Autodesk Inventor part; units mm, degrees
ref_plane "YZ Plane" through (0, 0, 0) normal (1, 0, 0) x (0, 1, 0)
ref_plane "XZ Plane" through (0, 0, 0) normal (0, 1, 0) x (-1, 0, 0)
ref_plane "XY Plane" through (0, 0, 0) normal (0, 0, 1) x (1, 0, 0)
sketch "Sketch1" plane through (0, 0, 0) normal (0, 0, 1) x (1, 0, 0)
  line L0 (-70, 0) -> (70, 0)
  line L1 (70, 0) -> (70, -400)
  line L2 (70, -400) -> (-70, -400)
  line L3 (-70, -400) -> (-70, 0)
  point P0 (0, 0)
  point P1 (0, 0)
  dimension "d0" = 140
  dimension "d1" = 400
extrude "Plate1" add sketch "Sketch1" along normal blind 2
sketch "Sketch2" plane through (72, -400, 2) normal (-1, 0, 0) x (0, -1, 0)
  line L0 (-400, 0) -> (0, 0)
  line L1 (0, 0) -> (0, -120)
  line L2 (0, -120) -> (-400, -120)
  line L3 (-400, -120) -> (-400, 0)
edge flange "Flange1" height 120 angle 90 thickness 2 bend radius 2.75 thickness toward (-1, 0, 0) relief round relief width 2 relief depth 1 edges at (70, -200, 0) wall of the first edge with corners at (72, 0, 2) (72, -400, 2) (72, -400, -118) (72, 0, -118)
bend "Bend1"
corner "Corner1"
sketch "Sketch3" plane through (-72, 0, 2) normal (1, 0, 0) x (0, 1, 0)
  line L0 (-400, 0) -> (0, 0)
  line L1 (0, 0) -> (0, -120)
  line L2 (0, -120) -> (-400, -120)
  line L3 (-400, -120) -> (-400, 0)
edge flange "Flange2" height 120 angle 90 thickness 2 bend radius 2.75 thickness toward (1, 0, 0) relief round relief width 2 relief depth 1 edges at (-70, -200, 0) wall of the first edge with corners at (-72, -400, 2) (-72, 0, 2) (-72, 0, -118) (-72, -400, -118)
bend "Bend2"
corner "Corner2"
sketch "Sketch4" plane through (70, 0, -120) normal (0, 0, 1) x (1, 0, 0)
  line L0 (0, -400) -> (0, 0)
  line L1 (0, 0) -> (25, 0)
  line L2 (25, 0) -> (25, -400)
  line L3 (25, -400) -> (0, -400)
edge flange "Flange3" height 25 angle 90 thickness 2 bend radius 2.75 thickness toward (0, 0, 1) relief round relief width 2 relief depth 1 edges at (72, -200, -118) wall of the first edge with corners at (70, -400, -120) (70, 0, -120) (95, 0, -120) (95, -400, -120)
bend "Bend3"
corner "Corner3"
sketch "Sketch5" plane through (-70, -400, -120) normal (0, 0, 1) x (1, 0, 0)
  line L0 (0, 400) -> (0, 0)
  line L1 (0, 0) -> (-25, 0)
  line L2 (-25, 0) -> (-25, 400)
  line L3 (-25, 400) -> (0, 400)
edge flange "Flange4" height 25 angle 90 thickness 2 bend radius 2.75 thickness toward (0, 0, 1) relief round relief width 2 relief depth 1 edges at (-72, -200, -118) wall of the first edge with corners at (-70, 0, -120) (-70, -400, -120) (-95, -400, -120) (-95, 0, -120)
bend "Bend4"
corner "Corner4"
sketch "Sketch6" plane through (95, -400, -118) normal (0, 0, 1) x (1, 0, 0)
  circle A0 centre (-10.125, 350) radius 4
  line L0 (-20.25, 400) -> (0, 400)
  point P0 (-95, 400)
  point P1 (-10.125, 400)
  dimension "d43" = 8
  dimension "d44" = 50
extrude "Extrusion1" cut sketch "Sketch6" against normal through all
pattern_linear "Rectangular Pattern2" count 4 spacing 100 along (0, -1, 0) count 2 spacing 169.75 along (-1, 0, 0) of "Extrusion1"
equation "\"d0\" = Ширина_крепления_корпуса"
equation "\"d1\" = Длина_базовой_пластины"
equation "\"d2\" = Thickness"
equation "\"d3\" = BendReliefWidth"
equation "\"d4\" = BendReliefDepth"
equation "\"d5\" = MinimumRemnant"
equation "\"d6\" = TransitionRadius"
equation "\"d7\" = Длина_крепления_корпуса"
equation "\"d9\" = BendRadius"
equation "\"d10\" = CornerReliefSize"
equation "\"d11\" = GapSize"
equation "\"d12\" = JacobiRadiusSize"
equation "\"d13\" = BendReliefWidth"
equation "\"d14\" = BendReliefDepth"
equation "\"d15\" = MinimumRemnant"
equation "\"d16\" = TransitionRadius"
equation "\"d17\" = Длина_крепления_корпуса"
equation "\"d19\" = BendRadius"
equation "\"d20\" = CornerReliefSize"
equation "\"d21\" = GapSize"
equation "\"d22\" = JacobiRadiusSize"
equation "\"d23\" = BendReliefWidth"
equation "\"d24\" = BendReliefDepth"
equation "\"d25\" = MinimumRemnant"
equation "\"d26\" = TransitionRadius"
equation "\"d29\" = BendRadius"
equation "\"d30\" = CornerReliefSize"
equation "\"d31\" = GapSize"
equation "\"d32\" = JacobiRadiusSize"
equation "\"d33\" = BendReliefWidth"
equation "\"d34\" = BendReliefDepth"
equation "\"d35\" = MinimumRemnant"
equation "\"d36\" = TransitionRadius"
equation "\"d39\" = BendRadius"
equation "\"d40\" = CornerReliefSize"
equation "\"d41\" = GapSize"
equation "\"d42\" = JacobiRadiusSize"
equation "\"BendReliefWidth\" = Thickness"
equation "\"BendReliefDepth\" = 0.5 * Thickness"
equation "\"CornerReliefSize\" = 4 * Thickness"
equation "\"MinimumRemnant\" = 2 * Thickness"
equation "\"TransitionRadius\" = BendRadius"
equation "\"JacobiRadiusSize\" = BendRadius"
equation "\"GapSize\" = Thickness"
properties part number "Кожух" material "Stainless Steel"
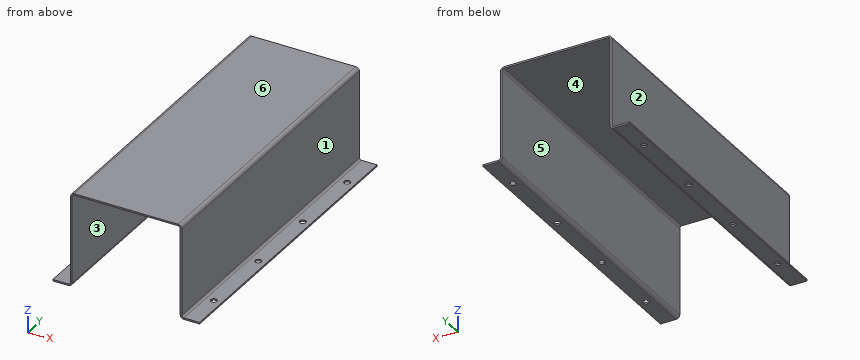
Part model, mm, in its own coordinate system. Face numbers are marked on the shaded views. A direction names the side the tool comes from. Coordinates: 2 decimals unless noted, no trailing zeros. Order: outer loops, then holes, each group sorted by start corner. A loop starts at its lowest first (then second) coordinate and runs counter-clockwise, first axis right, second up.
(1) Pull direction X, two halves, no side cores. Call the marked faces 1, 2, 3 and 4: pulls with the +X half, pulls with the -X half, needs draft (parallel to the pull), parting line crosses it, or undercut.
Check sheet entries:
face 1: pulls with the +X half
face 2: pulls with the -X half
face 3: undercut
face 4: undercut
(2) Slice it at B-B, the plane y = -150. Write the cut outline in (x, z) (3 decimals).
Check sheet entries:
outline: (-95, -120) - (-88.875, -120) - (-88.875, -118) - (-95, -118) - close; (-80.875, -120) - (-74.75, -120) arc R4.75 ccw to (-70, -115.25) - (-70, -2.75) arc R2.75 cw to (-67.25, 0) - (67.25, 0) arc R2.75 cw to (70, -2.75) - (70, -115.25) arc R4.75 ccw to (74.75, -120) - (80.875, -120) - (80.875, -118) - (74.75, -118) arc R2.75 cw to (72, -115.25) - (72, -2.75) arc R4.75 ccw to (67.25, 2) - (-67.25, 2) arc R4.75 ccw to (-72, -2.75) - (-72, -115.25) arc R2.75 cw to (-74.75, -118) - (-80.875, -118) - close; (88.875, -120) - (95, -120) - (95, -118) - (88.875, -118) - close
(3) Pin check, flat tips, straight feed: pin 1 Ø10 at (x, y) = (-88.5, -101.5) entering from +Z; pin 2 Ø1.5 at (x, y) = (-40, -120) entering from -Z; pin 3 Ø4 at (y, z) = (-337, -24.5) entering from -X. Stop position of each tip, or through.
Check sheet entries:
pin 1: stops at z = -118
pin 2: stops at z = 0
pin 3: stops at x = -72
(4) Probe L1, parallel to X at y = -118.5, z = -57; L2, parallel to X at y = -350, z = -118.6 (1 decimal); L3, parallel to Z at x = 5.5, y = -84. List the from-to ranges inside material, lowest first.
Check sheet entries:
L1: x = -72 to -70, 70 to 72
L2: x = -95 to -88.9, -80.9 to -71.4, 71.4 to 80.9, 88.9 to 95
L3: z = 0 to 2
(5) Tool access for the marked faces 5 and 6: list every direction of +Z, -Z, +X, -X, +Y, -Y with a clear straight run to the whole face (end or side of a thin tool).
Check sheet entries:
face 5: -Z, +Y, -Y
face 6: +Z, +X, -X, +Y, -Y
(6) Slice it at C-C, the plane y = -361.5. Write the cut outline in (x, z), and give its area (3 significant figures).
Check sheet entries:
outline: (-95, -120) - (-74.75, -120) arc R4.75 ccw to (-70, -115.25) - (-70, -2.75) arc R2.75 cw to (-67.25, 0) - (67.25, 0) arc R2.75 cw to (70, -2.75) - (70, -115.25) arc R4.75 ccw to (74.75, -120) - (95, -120) - (95, -118) - (74.75, -118) arc R2.75 cw to (72, -115.25) - (72, -2.75) arc R4.75 ccw to (67.25, 2) - (-67.25, 2) arc R4.75 ccw to (-72, -2.75) - (-72, -115.25) arc R2.75 cw to (-74.75, -118) - (-95, -118) - close
area: 847 mm2
(7) Slice it at A-A, the plane z = -98. Write the cut outline in (x, y).
Check sheet entries:
outline: (-72, -400) - (-70, -400) - (-70, 0) - (-72, 0) - close; (70, -400) - (72, -400) - (72, 0) - (70, 0) - close
(8) Slice it at D-D, the plane x = -25.5. Write the cut outline in (y, z), and give its area (3 significant figures).
Check sheet entries:
outline: (-400, 0) - (0, 0) - (0, 2) - (-400, 2) - close
area: 800 mm2
